Check sheet for the modelled part. Datum: model origin and axes. Units: mm. Round coordinates to 2 decimals unless told otherwise and drop trailing zeros. Put each result on its own line as item: value. Start each with the question number.
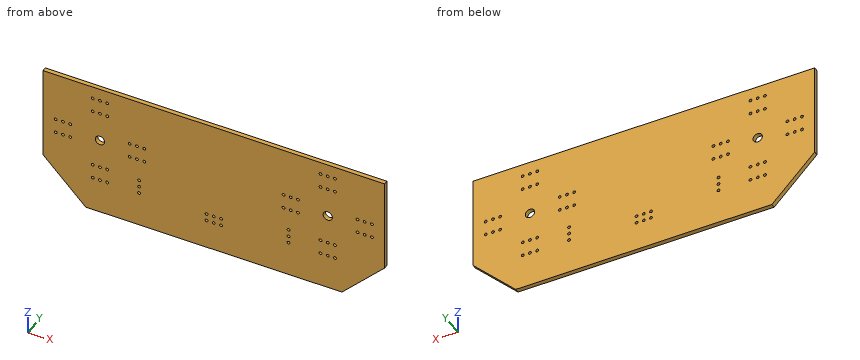
from build123d import *

# Parameters (mm, degrees)
SKETCH1_W           = 120
SKETCH1_H           = 48
BOSS_EXTRUDE1_DEPTH = 1.53
SKETCH2_R           = 0.5
SKETCH2_R_2         = 1.625
CUT_EXTRUDE1_DEPTH  = 67.229456437
SKETCH5_R           = 0.5
CUT_EXTRUDE2_DEPTH  = 67.229456437
CUT_EXTRUDE4_DEPTH  = 67.229456437
SKETCH7_R           = 0.5
CUT_EXTRUDE5_DEPTH  = 67.229456437


with BuildPart() as part:
    # Sketch1 → Boss-Extrude1 (new body)
    with BuildSketch(Plane(origin=(0, 0, 0), x_dir=(1, 0, 0), z_dir=(0, 1, 0))):
        with Locations((0, 4)):
            Rectangle(SKETCH1_W, SKETCH1_H)
    extrude(amount=BOSS_EXTRUDE1_DEPTH)

    # Sketch2 → Cut-Extrude1 (cut, through all)
    with BuildSketch(Plane(origin=(0, 1.53, 0), x_dir=(1, 0, 0), z_dir=(0, 1, 0))):
        with Locations(Location((-55.54, 2.54, 0), (0, 0, 270))):
            Circle(SKETCH2_R)
        with Locations(Location((-53, 2.54, 0), (0, 0, 270))):
            Circle(SKETCH2_R)
        with Locations(Location((-50.46, 2.54, 0), (0, 0, 270))):
            Circle(SKETCH2_R)
        with Locations(Location((-55.54, -2.54, 0), (0, 0, 270))):
            Circle(SKETCH2_R)
        with Locations(Location((-53, -2.54, 0), (0, 0, 270))):
            Circle(SKETCH2_R)
        with Locations(Location((-50.46, -2.54, 0), (0, 0, 270))):
            Circle(SKETCH2_R)
        with Locations(Location((-29.54, 2.54, 0), (0, 0, 270))):
            Circle(SKETCH2_R)
        with Locations(Location((-27, 2.54, 0), (0, 0, 270))):
            Circle(SKETCH2_R)
        with Locations(Location((-24.46, 2.54, 0), (0, 0, 270))):
            Circle(SKETCH2_R)
        with Locations(Location((-29.54, -2.54, 0), (0, 0, 270))):
            Circle(SKETCH2_R)
        with Locations(Location((-27, -2.54, 0), (0, 0, 270))):
            Circle(SKETCH2_R)
        with Locations(Location((-24.46, -2.54, 0), (0, 0, 270))):
            Circle(SKETCH2_R)
        with Locations(Location((-42.54, 15.54, 0), (0, 0, 270))):
            Circle(SKETCH2_R)
        with Locations(Location((-40, 15.54, 0), (0, 0, 270))):
            Circle(SKETCH2_R)
        with Locations(Location((-37.46, 15.54, 0), (0, 0, 270))):
            Circle(SKETCH2_R)
        with Locations(Location((-42.54, 10.46, 0), (0, 0, 270))):
            Circle(SKETCH2_R)
        with Locations(Location((-40, 10.46, 0), (0, 0, 270))):
            Circle(SKETCH2_R)
        with Locations(Location((-37.46, 10.46, 0), (0, 0, 270))):
            Circle(SKETCH2_R)
        with Locations(Location((-42.54, -10.46, 0), (0, 0, 270))):
            Circle(SKETCH2_R)
        with Locations(Location((-40, -10.46, 0), (0, 0, 270))):
            Circle(SKETCH2_R)
        with Locations(Location((-37.46, -10.46, 0), (0, 0, 270))):
            Circle(SKETCH2_R)
        with Locations(Location((-42.54, -15.54, 0), (0, 0, 270))):
            Circle(SKETCH2_R)
        with Locations(Location((-40, -15.54, 0), (0, 0, 270))):
            Circle(SKETCH2_R)
        with Locations(Location((-37.46, -15.54, 0), (0, 0, 270))):
            Circle(SKETCH2_R)
        with Locations(Location((-40, 0, 0), (0, 0, 270))):
            Circle(SKETCH2_R_2)
    cut_extrude1 = extrude(amount=-CUT_EXTRUDE1_DEPTH, mode=Mode.SUBTRACT)

    # Mirror1: Cut-Extrude1 across plane
    add(cut_extrude1.mirror(Plane(origin=(0, 0, 0), x_dir=(0, 0, 1), z_dir=(1, 0, 0))), mode=Mode.SUBTRACT)

    # Sketch5 → Cut-Extrude2 (cut, through all)
    with BuildSketch(Plane(origin=(0, 1.53, 0), x_dir=(1, 0, 0), z_dir=(0, 1, 0))):
        with Locations(Location((-2.54, 17.54, 0), (0, 0, 270))):
            Circle(SKETCH5_R)
        with Locations(Location((0, 17.54, 0), (0, 0, 270))):
            Circle(SKETCH5_R)
        with Locations(Location((2.54, 17.54, 0), (0, 0, 270))):
            Circle(SKETCH5_R)
        with Locations(Location((-2.54, 15, 0), (0, 0, 270))):
            Circle(SKETCH5_R)
        with Locations(Location((0, 15, 0), (0, 0, 270))):
            Circle(SKETCH5_R)
        with Locations(Location((2.54, 15, 0), (0, 0, 270))):
            Circle(SKETCH5_R)
    extrude(amount=-CUT_EXTRUDE2_DEPTH, mode=Mode.SUBTRACT)

    # Sketch6 → Cut-Extrude4 (cut, through all)
    with BuildSketch(Plane(origin=(0, 1.53, 0), x_dir=(1, 0, 0), z_dir=(0, 1, 0))):
        Polygon((-60, 28), (-45, 28), (-60, 13), align=None)
        Polygon((60, 28), (60, 13), (45, 28), align=None)
    extrude(amount=-CUT_EXTRUDE4_DEPTH, mode=Mode.SUBTRACT)

    # Sketch7 → Cut-Extrude5 (cut, through all)
    with BuildSketch(Plane(origin=(0, 1.53, 0), x_dir=(1, 0, 0), z_dir=(0, 1, 0))):
        with Locations(Location((-26.25, 15.54, 0), (0, 0, 270))):
            Circle(SKETCH7_R)
        with Locations(Location((-26.25, 13.02, 0), (0, 0, 270))):
            Circle(SKETCH7_R)
        with Locations(Location((-26.25, 10.5, 0), (0, 0, 270))):
            Circle(SKETCH7_R)
        with Locations(Location((26.25, 10.5, 0), (0, 0, 90))):
            Circle(SKETCH7_R)
        with Locations(Location((26.25, 13.02, 0), (0, 0, 90))):
            Circle(SKETCH7_R)
        with Locations(Location((26.25, 15.54, 0), (0, 0, 90))):
            Circle(SKETCH7_R)
    extrude(amount=-CUT_EXTRUDE5_DEPTH, mode=Mode.SUBTRACT)


solid = part.part
1. Gauge pin test, flat end, axial feed: P1, Ø4, axis at x = 40, z = 0, coming from the -Y side. Record the tip position at first contact, or that the pin passes through.
2. Material ranges on L1, parallel to Z at x = 29.54, y = 1.2; L2, parallel to Z at x = -37.46, y = 1.1; L3, parallel to X at y = 1.2, z = 0.5, recorded low to high. Write a range as [from, to].
3. Section check A-A, the plane y = 1.25. Give the number of separate pieces and of enclosed holes in the cut face, then the cut area to 3 significant figures.
Reply:
1. P1: stops at y = 0
2. L1: z = [-28, -3.04], [-2.04, 2.04], [3.04, 20]
2. L2: z = [-28, -16.04], [-15.04, -10.96], [-9.96, 9.96], [10.96, 15.04], [16.04, 20]
2. L3: x = [-60, -41.55], [-38.45, 38.45], [41.55, 60]
3. separate pieces: 1
3. enclosed holes: 62
3. area: 5,470 mm2
